The listing builds one solid part. Answer for the finished solid, in the listing's coordinates (mm). A direction names the side the tool comes from. Round coordinates to 2 decimals unless told otherwise and drop trailing zeros. Write each loop counter-clockwise with the first axis right and the second up, starting at its lowest first coordinate (ties: lowest second). Pieces come first, ordered by that corner, then holes. Notation, with made-up numbers: (37, -19) - (84, -19) arc R15 ccw to (84, -7) - close; hole circle Ø7 at (49.5, 37). An arc over 180 degrees is marked (long way). Use a Markdown table: item, result. Add a question column.
1) Each of these flat-tipped pins is pushed along its axis until it touches: P1, Ø1.5, axis at x = -1.5, y = 6, coming from the -Z side; P2, Ø1.6, axis at x = 0, z = 0, coming from the -Y side; P3, Ø1.5, axis at x = -2, y = 11, coming from the -Z side. Where does it stop, or does it pass through?
2) A cutting plane is placed at B-B (y = 5.75). Give the vertices of the cut face in (x, z).
3) A tool of negligible diameter and unlimited length cuts with its end or side. For faces 1 (the flat face through (0, 0.5, 0)), 2 (the cylindrical face through (-1.5, 6.75, -0.07)), 3 (the cylindrical face through (0.9, 0.39, 2.86)), from which of +Z, -Z, +X, -X, +Y, -Y can it reach the whole face along a straight path? Write none if from no direction.
4) A cutting plane is placed at C-C (z = 2). Give the vertices of the cut face in (x, y), then the cut area to 3 significant figures.
5) A cutting plane is placed at A-A (x = 0). Give the vertices of the cut face in (y, z), then the cut area to 3 significant figures.
6) A cutting plane is placed at D-D (x = 1.8). Give the vertices of the cut face in (y, z).
7) Find the intervals of material crossed by probe 1 along Y at (x, z) = (-2.35, -0.65); probe 2 along X at (y, z) = (8, -0.1); probe 3 along X at (y, z) = (5.5, -1.1), in increasing order. Write a range as from..to.
```python
from build123d import *

# Parameters (mm, degrees)
SKETCH_1_R          = 3
EXTRUDE_1_DEPTH     = 0.8
CUT_EXTRUDE_1_DEPTH = 0.5


# Read off the part's stored shape, not the designer's step: M3 机械螺纹 螺柱3
with BuildPart() as part:
    # 草图1 → 凸台-拉伸1 (new body)
    with BuildSketch(Plane(origin=(0, 0, 0), x_dir=(1, 0, 0), z_dir=(0, 1, 0))):
        with Locations(Location((0, 0, 0), (0, 0, 270))):
            Circle(SKETCH_1_R)
    extrude(amount=EXTRUDE_1_DEPTH)

    # M3 机械螺纹 螺柱3 outline → M3 机械螺纹 螺柱3 (revolve)
    with BuildSketch(Plane.XY):
        Polygon((1.2295, 12.8), (0, 12.8), (0, 0.8), (1.5, 0.8), (1.5, 12.5295), align=None)
    revolve(axis=Axis((0, 0, 0), (0, 1, 0)))

    # 草图8 → 切除-拉伸1 (cut)
    with BuildSketch(Plane.XZ):
        Polygon((1.154700538, 0), (0.577350269, 1), (-0.577350269, 1), (-1.154700538, 0), (-0.577350269, -1), (0.577350269, -1), align=None)
    extrude(amount=-CUT_EXTRUDE_1_DEPTH, mode=Mode.SUBTRACT)


solid = part.part
```
Entries:
| question | item | result |
|---|---|---|
| 1 | P1 | stops at z = -1.3 |
| 1 | P2 | stops at y = 0.5 |
| 1 | P3 | stops at z = -0.83 |
| 2 | outline | circle Ø3 at (0, 0) |
| 3 | face 1 | -Y |
| 3 | face 2 | +Y |
| 3 | face 3 | +Y, -Y |
| 4 | outline | (-2.24, 0) - (2.24, 0) - (2.24, 0.8) - (-2.24, 0.8) - close |
| 4 | area | 3.58 mm² |
| 5 | outline | (0, -3) - (0.8, -3) - (0.8, -1.5) - (12.53, -1.5) - (12.8, -1.23) - (12.8, 1.23) - (12.53, 1.5) - (0.8, 1.5) - (0.8, 3) - (0, 3) - (0, 1) - (0.5, 1) - (0.5, -1) - (0, -1) - close |
| 5 | area | 39.7 mm² |
| 6 | outline | (0, -2.4) - (0.8, -2.4) - (0.8, 2.4) - (0, 2.4) - close |
| 7 | probe 1 | y = 0..0.8 |
| 7 | probe 2 | x = -1.5..1.5 |
| 7 | probe 3 | x = -1.02..1.02 |
